from build123d import *

# Parameters (mm, degrees)
SKETCH1_W           = 20.32
SKETCH1_H           = 20
SKETCH1_R           = 1.25
BOSS_EXTRUDE1_DEPTH = 4


with BuildPart() as part:
    # Sketch1 → Boss-Extrude1 (new body)
    with BuildSketch(Plane(origin=(0, 4, 0), x_dir=(1, 0, 0), z_dir=(0, 1, 0))):
        with Locations((10.16, -10)):
            Rectangle(SKETCH1_W, SKETCH1_H)
        with Locations((6, -14.686)):
            Circle(SKETCH1_R, mode=Mode.SUBTRACT)
        with Locations((6, -5.314)):
            Circle(SKETCH1_R, mode=Mode.SUBTRACT)
        with BuildLine():
            Line((12.57, -12), (12.57, -8))
            ThreePointArc((12.57, -8), (15.32, -5.25), (18.07, -8))
            Line((18.07, -8), (18.07, -12))
            ThreePointArc((18.07, -12), (15.32, -14.75), (12.57, -12))
        make_face(mode=Mode.SUBTRACT)
    extrude(amount=-BOSS_EXTRUDE1_DEPTH)


solid = part.part
Verification items for the finished model (mm, model axes). A direction names the side the tool comes from. Coordinates: 2 decimals unless noted, no trailing zeros. Write each loop counter-clockwise with the first axis right and the second up, starting at its lowest first coordinate (ties: lowest second). Pieces come first, ordered by that corner, then holes. Notation, with made-up numbers: (12, 56.5) - (24, 56.5) arc R22 ccw to (24, 79.5) - close; hole circle Ø6 at (72, 40). An arc over 180 degrees is marked (long way). Answer as a JSON object with one key per item and string values.
(1) Tool access check on faces 4 (the flat face through (10, 4, 10)), 5 (the flat face through (18.07, 2, 10)). Record the directions out of +Z, -Z, +X, -X, +Y, -Y that give a thin tool (end or side, any length) a straight path to the whole face; none if there is none.
Report:
{"face 4": "+Z, -Z, +X, -X, +Y", "face 5": "+Y, -Y"}
(2) Cross-section at D-D on y = 3.25. Record the cut outline in (x, z).
Report:
{"outline": "(0, 0) - (20.32, 0) - (20.32, 20) - (0, 20) - close; hole circle Ø2.5 at (6, 5.31); hole circle Ø2.5 at (6, 14.69); hole (12.57, 8) arc R2.75 ccw to (18.07, 8) - (18.07, 12) arc R2.75 ccw to (12.57, 12) - close"}
(3) Mould release check, pull along Z, two halves, no side actions. Record for faces 1 (the flat face through (0, 2, 10)), 2 (the flat face through (10, 2, 20)), 3 (the flat face through (12.57, 2, 10)): pulls with the +Z half, pulls with the -Z half, needs draft (parallel to the pull), parting line crosses it, or undercut.
Report:
{"face 1": "needs draft", "face 2": "pulls with the +Z half", "face 3": "undercut"}
(4) Cross-section at B-B on z = 5. Record the cut outline in (x, y).
Report:
{"outline": "(0, 0) - (4.79, 0) - (4.79, 4) - (0, 4) - close; (7.21, 0) - (20.32, 0) - (20.32, 4) - (7.21, 4) - close"}
(5) Cross-section at A-A on x = 15.32. Record the cut outline in (y, z), plus the area to 3 significant figures.
Report:
{"outline": "(0, 0) - (4, 0) - (4, 5.25) - (0, 5.25) - close; (0, 14.75) - (4, 14.75) - (4, 20) - (0, 20) - close", "area": "42.0 mm^2"}
(6) Thickness scan on line 1 along Z through (x, y) = (6, 1.05); line 2 along X through (y, z) = (3.4, 9); line 3 along Z through (x, y) = (15, 2.05). Record the ranges inside material, lowest first.
Report:
{"line 1": "0 to 4.06, 6.56 to 13.44, 15.94 to 20", "line 2": "0 to 12.57, 18.07 to 20.32", "line 3": "0 to 5.27, 14.73 to 20"}
(7) Cross-section at C-C on x = 6. Record the cut outline in (y, z).
Report:
{"outline": "(0, 0) - (4, 0) - (4, 4.06) - (0, 4.06) - close; (0, 6.56) - (4, 6.56) - (4, 13.44) - (0, 13.44) - close; (0, 15.94) - (4, 15.94) - (4, 20) - (0, 20) - close"}
